Here's how the part is built. I have some questions about the finished solid (model axes, mm). Round coordinates to 2 decimals unless told otherwise and drop trailing zeros. Loops run counter-clockwise (first coordinate to the right, second up) from the corner with the lowest first, then second, coordinate; pieces in that order, holes last. Notation, with made-up numbers: (64.5, -38.75) -> (74.5, -38.75) arc R17 ccw to (74.5, -30.75) -> close; hole circle Ø10 at (-24.75, -0.75). An arc over 180 degrees is marked (long way). Use one line per item in the form item = value. Start each with the question number.
Item 1: I'm going to push flat-ended pins straight in: pin 1 Ø0.9 at (y, z) = (1.5, -33) entering from +X; pin 2 Ø0.9 at (y, z) = (1, 41) entering from -X; pin 3 Ø1.5 at (x, y) = (-2, 1) entering from +Z. Where does each tip first touch, or does it pass through?
Item 2: If we section it at B-B (y = 0.8): State how many separate pieces and enclosed holes the cut face has, then the cut area to 3 significant figures.
Item 3: If we section it at C-C (z = -32): Write out the boundary of the cut face in (x, y).
Item 4: If we section it at A-A (x = 22): Write out the boundary of the cut face in (y, z), then the cut area to 3 significant figures.
Item 5: If I drill on L1, parallel to Z at x = 22.5, y = 2.35; L2, parallel to X at y = 1.1, z = -22; L3, parallel to Z at x = 6.5, y = 2.6, over which ranges is the centre line in solid material (lowest first)? Write a range as [from, to].
Item 6: If we section it at D-D (x = -1.5): Write out the boundary of the cut face in (y, z), then the cut area to 3 significant figures.
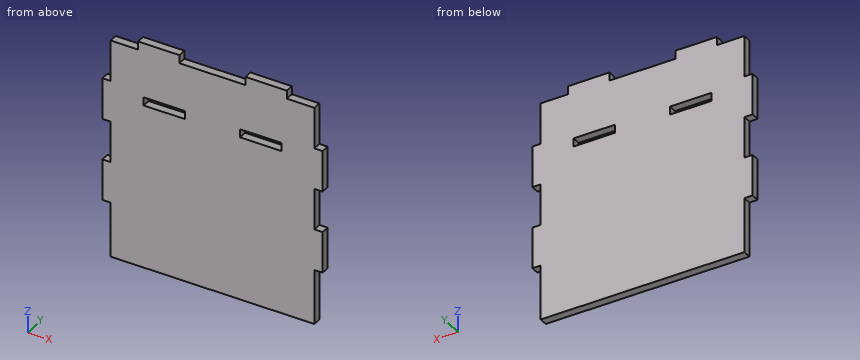
```python
from build123d import *

# Parameters (mm, degrees)
SKETCH_1_W          = 74
SKETCH_1_H          = 80
SKETCH_1_W_2        = 3
SKETCH_1_H_2        = 15
SKETCH_1_W_3        = 15
SKETCH_1_H_3        = 3
EXTRUDE_1_DEPTH     = 3
SKETCH_2_W          = 15
SKETCH_2_H          = 3
CUT_EXTRUDE_1_DEPTH = 3


with BuildPart() as part:
    # 草图1 → 凸台-拉伸1 (new body)
    with BuildSketch(Plane(origin=(0, 0, 0), x_dir=(1, 0, 0), z_dir=(0, 1, 0))):
        Rectangle(SKETCH_1_W, SKETCH_1_H)
        with Locations((-38.5, -17.5)):
            Rectangle(SKETCH_1_W_2, SKETCH_1_H_2)
        with Locations((-19.5, -41.5)):
            Rectangle(SKETCH_1_W_3, SKETCH_1_H_3)
        with Locations((19.5, -41.5)):
            Rectangle(SKETCH_1_W_3, SKETCH_1_H_3)
        with Locations((38.5, -17.5)):
            Rectangle(SKETCH_1_W_2, SKETCH_1_H_2)
        with Locations((38.5, 12.5)):
            Rectangle(SKETCH_1_W_2, SKETCH_1_H_2)
        with Locations((-38.5, 12.5)):
            Rectangle(SKETCH_1_W_2, SKETCH_1_H_2)
    extrude(amount=EXTRUDE_1_DEPTH)

    # 草图2 → 切除-拉伸1 (cut)
    with BuildSketch(Plane(origin=(0, 3, 0), x_dir=(1, 0, 0), z_dir=(0, 1, 0))):
        with Locations((-17.5, -21.5)):
            Rectangle(SKETCH_2_W, SKETCH_2_H)
        with Locations((17.5, -21.5)):
            Rectangle(SKETCH_2_W, SKETCH_2_H)
    extrude(amount=-CUT_EXTRUDE_1_DEPTH, mode=Mode.SUBTRACT)


solid = part.part
```
Values found:
q1.pin_1 = 37
q1.pin_2 = -27
q1.pin_3 = 40
q2.separate_pieces = 1
q2.enclosed_holes = 2
q2.area = 6,100 mm2
q3.outline = (-37, 0) -> (37, 0) -> (37, 3) -> (-37, 3) -> close
q4.outline = (0, -40) -> (3, -40) -> (3, 20) -> (0, 20) -> close; (0, 23) -> (3, 23) -> (3, 43) -> (0, 43) -> close
q4.area = 240 mm2
q5.L1 = [-40, 20], [23, 43]
q5.L2 = [-37, 37]
q5.L3 = [-40, 40]
q6.outline = (0, -40) -> (3, -40) -> (3, 40) -> (0, 40) -> close
q6.area = 240 mm2
